Geometry check sheet. Reference: the model listing, model coordinates, mm. A direction names the side the tool comes from. Round coordinates to 2 decimals unless told otherwise and drop trailing zeros. Write each loop counter-clockwise with the first axis right and the second up, starting at its lowest first coordinate (ties: lowest second). Pieces come first, ordered by that corner, then holes. Notation, with made-up numbers: M 37.5,-18 L 76.5,-18 A22 cw 76.5,20 Z; hole C 68,-25 d6. An arc over 180 degrees is marked long. Put each result on its own line as item: value. Start each with the question number.
(1) Mould release check, pull along X, two halves, no side actions. Record for faces 1 (the cylindrical face through (-9.28, 30.54, 46.62)), 2 (the flat face through (2, 33, 49)), 3 (the cylindrical face through (17.9, 30.04, 53.18)): pulls with the +X half, pulls with the -X half, needs draft (parallel to the pull), parting line crosses it, or undercut.
(2) Gauge pin test, flat ends, axial feed: pin 1 (5 mm diameter, centred on x = 5, z = 48.5, fed in from -Y); pin 2 (5 mm diameter, centred on x = 8, y = 28.5, fed in from -Z); pin 3 (2.5 mm diameter, centred on x = -13.5, z = 49, fed in from -Y). Record the tip position at first contact, or that the pin passes through.
(3) Section check D-D on x = 5. Record the cut outline in (y, z), then the cut area to 3 significant figures.
(4) Section check A-A on z = 48.75. Record the cut outline in (x, y).
(5) Section check B-B on x = -9. Record the cut outline in (y, z).
(6) Material ranges on probe 1 along X at (y, z) = (29.25, 48.75); probe 2 along X at (y, z) = (31.05, 48.75); probe 3 along X at (y, z) = (27.25, 51), recorded low to high.
(7) Tool access check on faces 4 (the flat face through (9, 31, 53.75)), 5 (the flat face through (2, 30, 49)), 6 (the flat face through (-11.652, 27, 49)). Record the directions out of +Z, -Z, +X, -X, +Y, -Y that give a thin tool (end or side, any length) a straight path to the whole face; none if there is none.
(8) Section check C-C on y = 31. Record the cut outline in (x, z).
Autodesk Inventor part; units mm, degrees
ref_plane "Work Plane1" through (-6, 33, 48.75) normal (0, 1, 0) x (0, 0, 1)
ref_plane "YZ Plane" through (0, 0, 0) normal (1, 0, 0) x (0, 1, 0)
ref_plane "XZ Plane" through (0, 0, 0) normal (0, 1, 0) x (-1, 0, 0)
ref_plane "Work Plane1" through (-6, 33, 48.75) normal (0, 1, 0) x (0, 0, 1)
sketch "Sketch1" plane through (-6, 33, 48.75) normal (0, 1, 0) x (0, 0, 1)
  arc A0 (5, 22.5) -> (3, 24.5) centre (3, 22.5) ccw
  line L0 (3, 24.5) -> (-3, 24.5)
  arc A1 (-3, 24.5) -> (-5, 22.5) centre (-3, 22.5) ccw
  line L1 (-5, 22.5) -> (-5, 14.5)
  line L2 (5, 14.5) -> (5, 22.5)
  line L3 (5, 4.5) -> (5, 14.5)
  line L4 (-5, 4.5) -> (-5, 14.5)
  line L5 (-5, 14.5) -> (5, 14.5)
  line L6 (5, -8) -> (-5, -8)
  line L7 (-5, 2) -> (-5, -8)
  line L8 (5, 2) -> (5, -8)
  line L9 (-5, 4.6724) -> (-5, 1.6802)
  line L10 (5, 1.6802) -> (5, 5.5636)
  point P0 (-48.75, 6)
extrude "Extrusion1" add sketch "Sketch1" against normal blind 3
sketch "Sketch2" plane through (-6, 30, 48.75) normal (0, -1, 0) x (1, 0, 0)
  line L0 (24.5, -3) -> (24.5, 3)
  arc A0 (24.5, 3) -> (22.5, 5) centre (22.5, 3) ccw
  line L1 (22.5, 5) -> (-8, 5)
  line L2 (-8, -5) -> (22.5, -5)
  arc A1 (22.5, -5) -> (24.5, -3) centre (22.5, -3) ccw
  line L3 (14.5, -5) -> (14.5, 5)
  point P0 (6, -48.75)
extrude "Extrusion2" add sketch "Sketch2" along normal blind 1.5
sketch "Sketch3" plane through (-6, 30, 48.75) normal (0, -1, 0) x (1, 0, 0)
  line L0 (-8, 5) -> (-8, -5)
  circle A0 centre (-3, 0) radius 2.15
  line L1 (2, 5) -> (-8, 5)
  line L2 (2, 5) -> (2, -5)
  line L3 (2, -5) -> (-8, -5)
  line L4 (-8, 5) -> (-8, -5)
  point P0 (6, -48.75)
extrude "Extrusion3" add sketch "Sketch3" along normal blind 2
sketch "Sketch4" plane through (-14, 33, 53.75) normal (0, 0, 1) x (1, 0, 0)
  line L0 (0, 0) -> (10, 0)
  line L1 (10, 0) -> (10, -5)
  line L2 (10, -5) -> (0, -5)
  line L3 (0, -5) -> (0, 0)
  point P0 (14, -33)
extrude "Extrusion4" add sketch "Sketch4" along normal blind 2
sketch "Sketch5" plane through (16.5, 33, 43.75) normal (0, 0, -1) x (-1, 0, 0)
  line L0 (30.5, -5) -> (20.5, -5)
  line L1 (30.5, 0) -> (30.5, -5)
  line L2 (30.5, 0) -> (20.5, 0)
  line L3 (20.5, 0) -> (20.5, -5)
  line L4 (20.5, -5) -> (30.5, -5)
  line L5 (30.5, -5) -> (30.5, 0)
  point P0 (16.5, -33)
extrude "Extrusion5" add sketch "Sketch5" along normal blind 2
sketch "Sketch6" plane through (-6, 33, 48.75) normal (0, 1, 0) x (1, 0, 0)
  circle A0 centre (-3, 0) radius 2.15
  point P0 (6, 48.75)
extrude "Extrusion6" cut sketch "Sketch6" against normal up to next
sketch "Sketch7" plane through (-6, 28, 48.75) normal (0, -1, 0) x (1, 0, 0)
  line L0 (-8, -7) -> (-8, 7)
  line L1 (2, -7) -> (-8, -7)
  line L2 (2, 7) -> (2, -7)
  line L3 (-8, 7) -> (2, 7)
  line L4 (2, -5) -> (-8, -5)
  line L5 (2, 5) -> (-8, 5)
  point P0 (6, -48.75)
extrude "Extrusion7" add sketch "Sketch7" along normal blind 4 contours L0 L4 L2 L1 | L0 L3 L2 L5
sketch "Sketch8" plane through (-14, 28, 43.75) normal (0, 0, 1) x (1, 0, 0)
  line L0 (0, 0) -> (10, 0)
  line L1 (0, 0) -> (0, -4)
  line L2 (10, -4) -> (0, -4)
  line L3 (10, 0) -> (10, -4)
  point P0 (14, -28)
extrude "Extrusion8" cut sketch "Sketch8" against normal blind 0.3
sketch "Sketch9" plane through (-4, 28, 53.75) normal (0, 0, -1) x (-1, 0, 0)
  line L0 (0, 0) -> (10, 0)
  line L1 (0, 0) -> (0, -4)
  line L2 (10, -4) -> (0, -4)
  line L3 (10, 0) -> (10, -4)
  point P0 (-4, -28)
extrude "Extrusion9" cut sketch "Sketch9" against normal blind 0.3
sketch "Sketch10" plane through (-6, 28.5, 48.75) normal (0, -1, 0) x (1, 0, 0)
  line L0 (24.5, -3) -> (24.5, 3)
  arc A0 (24.5, 3) -> (22.5, 5) centre (22.5, 3) ccw
  line L1 (22.5, 5) -> (14.5, 5)
  line L2 (14.5, 5) -> (14.5, -5)
  line L3 (14.5, -5) -> (22.5, -5)
  arc A1 (22.5, -5) -> (24.5, -3) centre (22.5, -3) ccw
  point P0 (6, -48.75)
extrude "Extrusion10" add sketch "Sketch10" along normal blind 1.5
sketch "Sketch11" plane through (-6, 28, 48.75) normal (0, -1, 0) x (1, 0, 0)
  line L0 (-8, -5.3) -> (-8, 5.3)
  line L1 (-8, -5.3) -> (2, -5.3)
  line L2 (-8, 5.3) -> (-5.652, 5.3)
  line L3 (-5.652, 5.3) -> (-5.652, -5.3)
  line L4 (-5.652, -5.3) -> (-8, -5.3)
  line L5 (-8, -5.3) -> (-8, 5.3)
  point P0 (6, -48.75)
extrude "Extrusion11" add sketch "Sketch11" along normal blind 2.6
properties part number "CradleTop"
Answers follow:
1. face 1: undercut
1. face 2: needs draft
1. face 3: pulls with the +X half
2. pin 1: stops at y = 30
2. pin 2: stops at z = 43.75
2. pin 3: stops at y = 25.4
3. outline: M 30,43.75 L 33,43.75 L 33,53.75 L 30,53.75 Z
3. area: 30.0 mm^2
4. outline: M -14,25.4 L -11.65,25.4 L -11.65,28 L -11.15,28 L -11.15,33 L -14,33 Z; M -6.85,28 L -4,28 L -4,30 L 8.5,30 L 8.5,27 L 18.5,27 L 18.5,33 L -6.85,33 Z
5. outline: M 24,41.75 L 33,41.75 L 33,46.6 L 28,46.6 L 28,43.45 L 24,43.45 Z; M 24,54.05 L 28,54.05 L 28,50.9 L 33,50.9 L 33,55.75 L 24,55.75 Z
6. probe 1: x = -14 to -11.15, -6.85 to -4, 8.5 to 18.5
6. probe 2: x = -14 to -11.15, -6.85 to 18.5
6. probe 3: x = -14 to -11.65, 8.5 to 18.5
7. face 4: +Z, +X, +Y, -Y
7. face 5: +Z, -Z, -Y
7. face 6: -Y
8. outline: M -14,41.75 L -4,41.75 L -4,43.75 L 16.5,43.75 A2 ccw 18.5,45.75 L 18.5,51.75 A2 ccw 16.5,53.75 L -4,53.75 L -4,55.75 L -14,55.75 Z; hole C -9,48.75 d4.3
